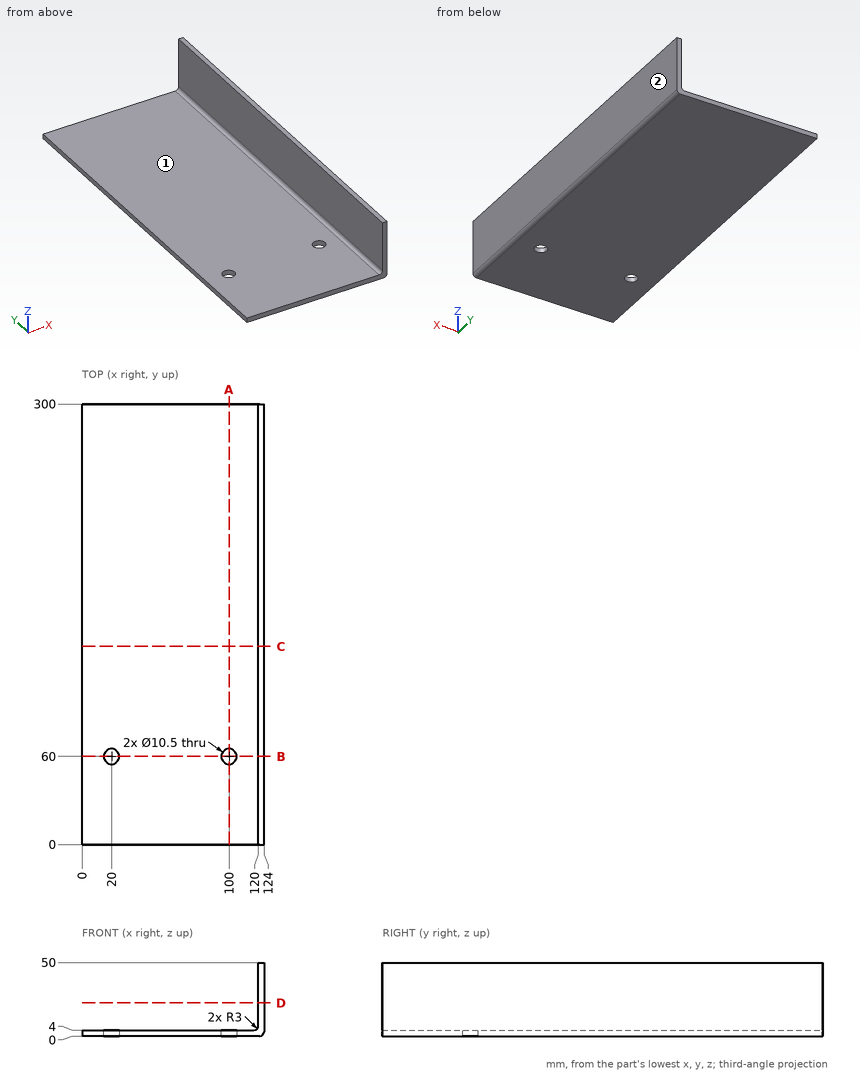
Answer from the drawing. Dimensions are ordinates in mm from the lowest x, y and z of the part. A direction names the side the tool comes from. Give positions to 0.01 mm unless a question says otherwise; leave off trailing zeros. Write each loop counter-clockwise with the first axis right and the second up, starting at its lowest first coordinate (ties: lowest second). Pieces come first, ordered by that corner, then holes.
1) Section A-A (x = 100) is taken. Write down the section's boundary in (y, z).
2) Section C-C (y = 135) is taken. Write down the section's boundary in (x, z).
3) Find the intervals of material crossed by L1, parallel to Y at x = 20, z = 3.05; L2, parallel to X at y = 193.5, z = 22.5; L3, parallel to Z at x = 72, y = 208, in increasing order.
4) Section B-B (y = 60) is taken. Write down the section's boundary in (x, z).
5) Section D-D (z = 22.5) is taken. Write down the section's boundary in (x, y).
6) A tool of negligible diameter and unlimited length cuts with its end or side. For the marked faces 1 and 2, from which of +Z, -Z, +X, -X, +Y, -Y can it reach the whole face along a straight path? Write none if from no direction.
7) Given P1, Ø3, axis at x = 59.5, y = 153, coming from the +Z side; P2, Ø21.5, axis at y = 190.5, z = 35, coming from the -X side, each flat-ended and moving along its own axis, determine where each tip first touches the part or whether it passes through.
Response:
1. outline: (0, 0) - (54.75, 0) - (54.75, 4) - (0, 4) - close; (65.25, 0) - (300, 0) - (300, 4) - (65.25, 4) - close
2. outline: (0, 0) - (121, 0) arc R3 ccw to (124, 3) - (124, 50) - (120, 50) - (120, 7) arc R3 cw to (117, 4) - (0, 4) - close
3. L1: y = 0 to 54.75, 65.25 to 300
3. L2: x = 120 to 124
3. L3: z = 0 to 4
4. outline: (0, 0) - (14.75, 0) - (14.75, 4) - (0, 4) - close; (25.25, 0) - (94.75, 0) - (94.75, 4) - (25.25, 4) - close; (105.25, 0) - (121, 0) arc R3 ccw to (124, 3) - (124, 50) - (120, 50) - (120, 7) arc R3 cw to (117, 4) - (105.25, 4) - close
5. outline: (120, 0) - (124, 0) - (124, 300) - (120, 300) - close
6. face 1: +Z, -X, +Y, -Y
6. face 2: +Z, -Z, +X, +Y, -Y
7. P1: stops at z = 4
7. P2: stops at x = 120
